The listing builds one solid part. Answer for the finished solid, in the listing's coordinates (mm). Give positions to 0.01 mm unless a question says otherwise; leave off trailing zeros. Write each loop counter-clockwise with the first axis right and the second up, starting at its lowest first coordinate (ties: lowest second). Pieces come first, ordered by that corner, then holes. Notation, with made-up numbers: (56.25, 18.5) - (110.25, 18.5) arc R22 cw to (110.25, 54.5) - close; hole circle Ø3 at (63, -10.5). An arc over 180 degrees is marked (long way). Write each question's results on one line, items separated by ' | '. Start each with the question number.
Q1. Section B-B (y = 512) is taken. Determine the outline of the cut face in (x, z).
Q2. Section C-C (z = 28) is taken. Determine the outline of the cut face in (x, y).
Q3. Section A-A (x = 494.5) is taken. Determine the outline of the cut face in (y, z).
Q4. Flat-ended cylindrical pins translate along their axes: pin 1 Ø8 at (x, z) = (827, -169) entering from +Y; pin 2 Ø4 at (x, z) = (465.5, 237.5) entering from +Y; pin 3 Ø1 at (x, z) = (782.5, -101) entering from +Y. Find the tip coordinate at first contact, or state that the pin passes through.
Q5. Find the intervals of material crossed by probe 1 along X at (y, z) = (348, -40); probe 2 along Y at (x, z) = (993, -273); probe 3 along Y at (x, z) = (644.5, -66), in increasing order.
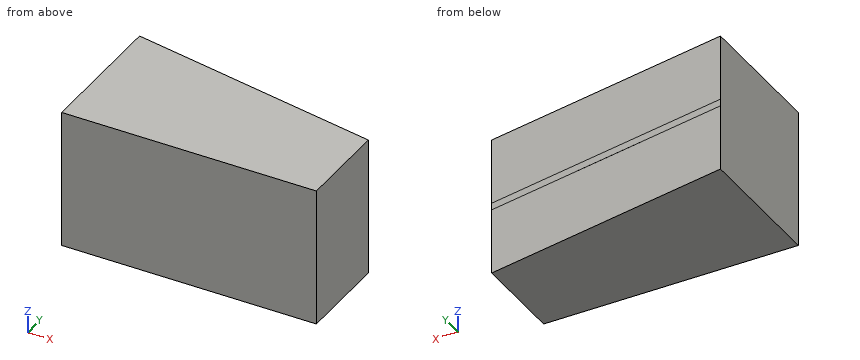
Autodesk Inventor part; units mm, degrees
ref_plane "YZ Plane" through (0, 0, 0) normal (1, 0, 0) x (0, 1, 0)
ref_plane "XZ Plane" through (0, 0, 0) normal (0, 1, 0) x (-1, 0, 0)
ref_plane "XY Plane" through (0, 0, 0) normal (0, 0, 1) x (1, 0, 0)
sketch "スケッチ1" plane through (0, 0, 0) normal (0, 0, 1) x (1, 0, 0)
  line L0 (0, 0) -> (1100, 0)
  line L1 (1100, 0) -> (1100, 400)
  line L2 (1100, 400) -> (0, 600)
  line L3 (0, 600) -> (0, 0)
  dimension "d0" = 600
  dimension "d1" = 1100
  dimension "d2" = 400
extrude "押し出し1" add sketch "スケッチ1" along normal mid plane 600
sketch "スケッチ2" plane through (0, 0, 0) normal (0, 0, 1) x (1, 0, 0)
  line L0 (1100, 400) -> (0, 600)
  line L1 (0, 600) -> (0, 600.1016)
  line L2 (0, 600.1016) -> (1100.0179, 400.0984)
  line L3 (1100.0179, 400.0984) -> (1100, 400)
  point P0 (0, 0)
  dimension "d5" = 0.1
extrude "押し出し2" add sketch "スケッチ2" along normal mid plane 30
properties part number "Slope 3"
Answers below:
1) outline: (0, -300) - (484, -300) - (484, -15) - (484.56, -15) - (484.56, 15) - (484, 15) - (484, 300) - (0, 300) - close
2) outline: (0, 0) - (1100, 0) - (1100, 400) - (0, 600) - close
3) outline: (0, -300) - (510.09, -300) - (510.09, -15) - (510.19, -15) - (510.19, 15) - (510.09, 15) - (510.09, 300) - (0, 300) - close
4) pin 1: stops at y = 450.36 | pin 2: stops at y = 515.73 | pin 3: stops at y = 457.82
5) probe 1: x = 0 to 1100 | probe 2: y = 0 to 419.45 | probe 3: y = 0 to 482.82
